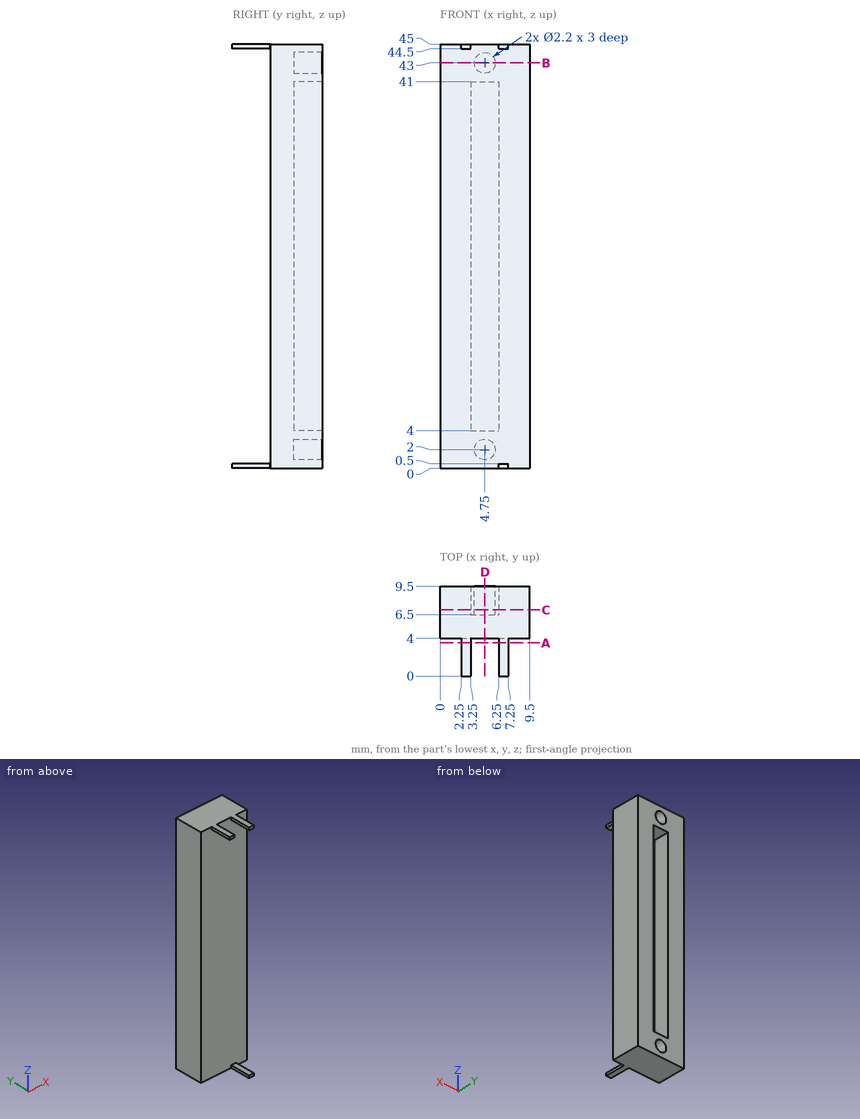
Input: dimensioned drawing with shaded views. Units: mm. Origin: part minimum x, y, z. Round coordinates to 2 decimals unless told otherwise and drop trailing zeros. Order: outer loops, then holes, each group sorted by start corner. A loop starts at its lowest first (then second) coordinate and runs counter-clockwise, first axis right, second up. Notation, with made-up numbers: (-16.75, -37) - (14.25, -37) arc R15 ccw to (14.25, -19) - close; hole circle Ø8 at (3, 76.5). An arc over 180 degrees is marked (long way). Use CSV: the item, a comma, the result in double quotes. Start each with the question number.
Q1. Material intervals for line 1 along X through (y, z) = (7, 9); line 2 along X through (y, z) = (8.65, 2); line 3 along Y through (x, z) = (0.75, 20), sorted ascending. Write a range as from..to.
Q2. Section query B-B (z = 43). Return loops of the section in (x, y), and give its area (4 significant figures).
Q3. Section query A-A (y = 3.5). Return loops of the section in (x, z), and give its area (3 significant figures).
Q4. Section query D-D (x = 4.75). Return loops of the section in (y, z), and give its area (3 significant figures).
Q5. First-contact query: pin 1 (1.1 mm diameter, centred on x = 5, z = 2, fed in from +Y); pin 2 (5 mm diameter, centred on x = 6, z = 20.5, fed in from -Y); pin 3 (0.6 mm diameter, centred on y = 2, z = 44.5, fed in from -X). Flat tips, straight axial feed; report the tip coordinate or a pass-through.
Q6. Section query C-C (y = 7). Return loops of the section in (x, z).
Result set:
1,line 1,"x = 0..3.25, 6.25..9.5"
1,line 2,"x = 0..3.65, 5.85..9.5"
1,line 3,"y = 4..9.5"
2,outline,"(0, 4) - (9.5, 4) - (9.5, 9.5) - (5.85, 9.5) - (5.85, 6.5) - (3.65, 6.5) - (3.65, 9.5) - (0, 9.5) - close"
2,area,"45.65 mm2"
3,outline,"(2.25, 44.5) - (3.25, 44.5) - (3.25, 45) - (2.25, 45) - close; (6.25, 0) - (7.25, 0) - (7.25, 0.5) - (6.25, 0.5) - close; (6.25, 44.5) - (7.25, 44.5) - (7.25, 45) - (6.25, 45) - close"
3,area,"1.50 mm2"
4,outline,"(4, 0) - (9.5, 0) - (9.5, 0.9) - (6.5, 0.9) - (6.5, 3.1) - (9.5, 3.1) - (9.5, 4) - (6.5, 4) - (6.5, 41) - (9.5, 41) - (9.5, 41.9) - (6.5, 41.9) - (6.5, 44.1) - (9.5, 44.1) - (9.5, 45) - (4, 45) - close"
4,area,"123 mm2"
5,pin 1,"stops at y = 6.5"
5,pin 2,"stops at y = 4"
5,pin 3,"stops at x = 2.25"
6,outline,"(0, 0) - (9.5, 0) - (9.5, 45) - (0, 45) - close; hole (3.25, 4) - (6.25, 4) - (6.25, 41) - (3.25, 41) - close; hole circle Ø2.2 at (4.75, 2); hole circle Ø2.2 at (4.75, 43)"
